Design review of the part built by this model. Coordinates are the model's own, in mm. A direction names the side the tool comes from. Round coordinates to 2 decimals unless told otherwise and drop trailing zeros. Order: outer loops, then holes, each group sorted by start corner. A loop starts at its lowest first (then second) coordinate and runs counter-clockwise, first axis right, second up. Notation, with made-up numbers: (-26, 1.5) - (-18, 1.5) arc R17 cw to (-18, 33.5) - close; hole circle Ø1 at (43.5, -13). An arc over 180 degrees is marked (long way). Use CSV: the item, a comma, the result in double quotes.
from build123d import *

# Parameters (mm, degrees)
F2_W     = 88.9
F2_H     = 15.875
F3_DEPTH = 31.75
F4_SIZE  = 6.35
F5_R     = 18.161
F6_DEPTH = 60.326
F7_SIZE  = 1.27


with BuildPart() as f1:
    # F0 (on Front) → F1 (revolve)
    with BuildSketch(Plane.XZ):
        with BuildLine():
            Line((-254, 0), (0, 0))
            Line((0, 0), (0, 17.4625))
            ThreePointArc((0, 17.4625), (-5.487017, 25.425187), (-12.801965, 31.75))
            Line((-12.801965, 31.75), (-234.95, 31.75))
            Line((-234.95, 31.75), (-234.95, 44.45))
            Line((-234.95, 44.45), (-254, 44.45))
            Line((-254, 44.45), (-254, 0))
        make_face()
    revolve(axis=Axis((-125.804233, 0, 0), (-1, 0, 0)))

    # F2 (on Top) → F3 (cut, symmetric)
    with BuildSketch(Plane.XY):
        with Locations((-44.45, 23.8125)):
            Rectangle(F2_W, F2_H)
        with Locations((-44.45, -23.8125)):
            Rectangle(F2_W, F2_H)
    extrude(amount=F3_DEPTH, both=True, mode=Mode.SUBTRACT)

    # F4
    f4_edges = [f1.edges().sort_by_distance(p)[0] for p in [
        (-88.9, -15.875, 0),
        (-88.9, 15.875, 0),
    ]]
    chamfer(f4_edges, length=F4_SIZE)

    # F5 (on face) → F6 (cut, through all)
    with BuildSketch(Plane.XZ.offset(15.875)):
        with Locations((-31.75, 0)):
            Circle(F5_R)
    extrude(amount=-F6_DEPTH, mode=Mode.SUBTRACT)

    # F7
    f7_edges = [f1.edges().sort_by_distance(p)[0] for p in [
        (-234.95, 0, -44.45),
        (-254, 0, -44.45),
    ]]
    chamfer(f7_edges, length=F7_SIZE)


solid = f1.part
1) We need section A-A (z = 0). Give the boundary of the cut face in (x, y) (3 decimals).
Data:
outline,"(-254, -43.18) - (-252.73, -44.45) - (-236.22, -44.45) - (-234.95, -43.18) - (-234.95, -31.75) - (-88.9, -31.75) - (-88.9, -22.225) - (-82.55, -15.875) - (-49.911, -15.875) - (-49.911, 15.875) - (-82.55, 15.875) - (-88.9, 22.225) - (-88.9, 31.75) - (-234.95, 31.75) - (-234.95, 43.18) - (-236.22, 44.45) - (-252.73, 44.45) - (-254, 43.18) - close; (-13.589, -15.875) - (0, -15.875) - (0, 15.875) - (-13.589, 15.875) - close"
2) To check wall thickness, follow L1, parallel to Z at x = -31.75, y = -1.5; L2, parallel to Z at x = -25.5, y = 7.5; L3, parallel to X at y = -12, z = -38. State the ranges of each line that lie inside material, in increasing order. Write a range as from..to.
Data:
L1,"z = -31.71..-18.16, 18.16..31.71"
L2,"z = -30.85..-17.05, 17.05..30.85"
L3,"x = -254..-234.95"
3) Insertion check: pin 1 Ø12 at (x, z) = (-47.5, -26.5) entering from +Y (3 decimals); pin 2 Ø5 at (x, y) = (-179.5, 12) entering from -Z; pin 3 Ø8 at (x, y) = (-106, -9.5) entering from -Z. Each pin has a flat end and moves straight along its axis. Give the tip position at first contact, or say it passes through.
Data:
pin 1,"stops at y = 15.875"
pin 2,"stops at z = -30.3"
pin 3,"stops at z = -31.27"
4) The part is to be moulded in two halves that separate along X. For faces 1 (the face through (0, 0, 0)), 2 (the face through (-254, 1, -1)), 3 (the face through (-51, 15.875, 0)), 4 (the face through (-45.14, -0.22, 12.27)), say which applies: +X half, -X half, draft (parallel to the pull), parting line (faces both ways), or undercut.
Data:
face 1,"+X half"
face 2,"-X half"
face 3,"draft"
face 4,"undercut"
5) We need section C-C (x = -170). Give the boundary of the cut face in (y, z), then the cut area to 3 significant figures.
Data:
outline,"circle Ø63.5 at (0, 0)"
area,"3,170 mm2"
6) We need section B-B (x = -31.75). Give the boundary of the cut face in (y, z) (3 decimals), then the cut area to 3 significant figures.
Data:
outline,"(-15.875, -27.496) arc R31.75 ccw to (15.875, -27.496) - (15.875, -18.161) - (-15.875, -18.161) - close; (-15.875, 18.161) - (15.875, 18.161) - (15.875, 27.496) arc R31.75 ccw to (-15.875, 27.496) - close"
area,"775 mm2"
7) For faces 5 (the face through (-234.95, 23, 23)), 6 (the face through (-51, -15.875, 0)), 7 (the face through (-88.9, 26, 0)), list the 3-axis set-ups (+Z, -Z, +X, -X, +Y, -Y) from which the entire face can be reached by the end or side of a thin tool; tool diameter is ignored.
Data:
face 5,"+X"
face 6,"+Z, -Z, +X, -Y"
face 7,"+Z, -Z, +X, +Y"
